```python
from build123d import *

# Parameters (mm, degrees)
PAD_DEPTH      = 360
PAD_DEPTH_BACK = 360
SKETCH001_R    = 271.855749
PAD001_DEPTH   = 100
SKETCH002_R    = 205.042507
POCKET_DEPTH   = 50
SKETCH003_W    = 782.000423
SKETCH003_H    = 725.272034
PAD002_DEPTH   = 100
SKETCH004_R    = 29.312065
SKETCH004_R_2  = 31.24981
SKETCH004_W    = 72.380981
SKETCH004_H    = 260.571579
SKETCH004_W_2  = 73.828552
SKETCH004_H_2  = 112.914345
PAD003_DEPTH   = 2


with BuildPart() as part:
    # Sketch → Pad (new body, two sides)
    with BuildSketch(Plane.YZ) as pad_sk:
        with BuildLine():
            Line((0, 0), (720, 0))
            ThreePointArc((720, 0), (770.07692, 500), (720, 1000))
            Line((0, 1000), (720, 1000))
            ThreePointArc((0, 1000), (-51.829558, 500), (0, 0))
        make_face()
    extrude(amount=PAD_DEPTH)
    extrude(pad_sk.sketch, amount=-PAD_DEPTH_BACK)

    # Sketch001 → Pad001 (join)
    with BuildSketch(Plane.XZ):
        with Locations((10.953636, 519.742493)):
            Circle(SKETCH001_R)
    extrude(amount=PAD001_DEPTH)

    # Sketch002 (on Face8 of Pad001) → Pocket (cut)
    with BuildSketch(Plane(origin=(0, -100, 0), x_dir=(0, 0, -1), z_dir=(0, -1, 0))):
        with Locations((-514.021362, 4.681509)):
            Circle(SKETCH002_R)
    extrude(amount=-POCKET_DEPTH, mode=Mode.SUBTRACT)

    # Sketch003 (on Face2 of Pocket) → Pad002 (join)
    with BuildSketch(Plane(origin=(0, 0, 1000), x_dir=(0, -1, 0), z_dir=(0, 0, 1))):
        with Locations((-353.783052, -1.157959)):
            Rectangle(SKETCH003_W, SKETCH003_H)
    extrude(amount=-PAD002_DEPTH)

    # Sketch004 (on Face4 of Pad002) → Pad003 (join)
    with BuildSketch(Plane(origin=(0, -37.217159, 0), x_dir=(0, 0, -1), z_dir=(0, -1, 0))):
        with Locations((-942.983643, -255.463287)):
            Circle(SKETCH004_R)
        with Locations((-940.088379, -143.996552)):
            Circle(SKETCH004_R_2)
        with Locations((-950.22174, 209.222724)):
            Rectangle(SKETCH004_W, SKETCH004_H)
        with Locations((-952.393158, -19.501239)):
            Rectangle(SKETCH004_W_2, SKETCH004_H_2)
    extrude(amount=PAD003_DEPTH)


solid = part.part
```
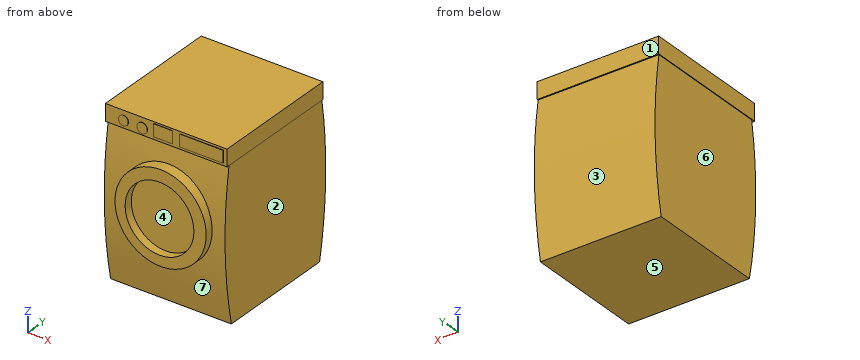
The listing builds one solid part. Answer for the finished solid, in the listing's coordinates (mm). Face numbers are marked on the shaded views. A direction names the side the tool comes from. Coordinates: 2 decimals unless noted, no trailing zeros. Write each loop counter-clockwise with the first axis right and the second up, starting at its lowest first coordinate (ties: lowest second). Pieces come first, ordered by that corner, then holes. Notation, with made-up numbers: M 55,76.25 L 65,76.25 A31 ccw 65,108.25 Z; hole C 55.5,26.5 d7. An arc over 180 degrees is marked long. Use a Markdown table: item, result. Add a question column.
1. Section D-D (z = 163.5) is taken. Give the vertices of the cut face in (x, y), plus the area to 3 significant figures.
2. Section B-B (x = 123.5) is taken. Give the vertices of the cut face in (y, z).
3. Section C-C (x = 21.5) is taken. Give the vertices of the cut face in (y, z), plus the area to 3 significant figures.
4. Which of the six approach directions +Z, -Z, +X, -X, +Y, -Y give full straight-line access (tool end or side, diameter ignored) to the marked faces 1, 2 and 3?
5. Straight lines are drawn through the part: line 1 along X through (y, z) = (298, 601.5); line 2 along Y through (x, z) = (225.5, 921.5); line 3 along Y through (x, z) = (-293, 211.5). For each, find the intervals that lie inside material, in ascending order. Write a range as [from, to].
6. For a pull along Z with two mould halves and no side action, classify the marked faces 4, 5, 6 and 7 as +Z half, -Z half, draft (parallel to the pull), parting line (faces both ways), or undercut.
7. Given P1, Ø1.6, axis at y = -38.5, z = 940.5, coming from the -X side; P2, Ø18.5, axis at x = -149.5, z = 942, coming from the -Y side; P3, Ø1.5, axis at x = -278.5, z = 174.5, coming from the -Y side, each flat-ended and moving along its own axis, determine where each tip first touches the part or whether it passes through.
8. Section A-A (z = 539) is taken. Give the vertices of the cut face in (x, y).
Data:
| question | item | result |
|---|---|---|
| 1 | outline | M -360,-28.49 L 360,-28.49 L 360,747.52 L -360,747.52 Z |
| 1 | area | 559,000 mm2 |
| 2 | outline | M -100,272.28 L -41.17,272.28 A2437.67 ccw 0,0 L 720,0 A2521.2 ccw 738.14,900 L 744.78,900 L 744.78,1000 L -37.22,1000 L -37.22,986.41 L -39.22,986.41 L -39.22,914.03 L -37.22,914.03 L -37.22,900 L -18.79,900 A2437.67 ccw -37.14,767.21 L -100,767.21 L -100,681.13 L -50,681.13 L -50,346.91 L -100,346.91 Z |
| 3 | outline | M -100,248.09 L -38.78,248.09 A2437.67 ccw 0,0 L 720,0 A2521.2 ccw 738.14,900 L 744.78,900 L 744.78,1000 L -37.22,1000 L -37.22,989.31 L -39.22,989.31 L -39.22,915.48 L -37.22,915.48 L -37.22,900 L -18.79,900 A2437.67 ccw -34.35,791.39 L -100,791.39 L -100,718.37 L -50,718.37 L -50,309.67 L -100,309.67 Z |
| 3 | area | 801,000 mm2 |
| 4 | face 1 | +Z, +X, -X, +Y |
| 4 | face 2 | -Z, +X, +Y, -Y |
| 4 | face 3 | +X, -X, +Y |
| 5 | line 1 | x = [-360, 360] |
| 5 | line 2 | y = [-39.22, 744.78] |
| 5 | line 3 | y = [-34.7, 753.52] |
| 6 | face 4 | undercut |
| 6 | face 5 | -Z half |
| 6 | face 6 | draft |
| 6 | face 7 | undercut |
| 7 | P1 | stops at x = -284.73 |
| 7 | P2 | stops at y = -39.22 |
| 7 | P3 | stops at y = -30.1 |
| 8 | outline | M -360,-51.52 L -260.22,-51.52 L -260.22,-100 L -198.83,-100 L -198.83,-50 L 208.2,-50 L 208.2,-100 L 282.13,-100 L 282.13,-51.52 L 360,-51.52 L 360,769.78 L -360,769.78 Z |
